Here's how the part is built. I have some questions about the finished solid (model axes, mm). Face numbers are marked on the shaded views. A direction names the side the tool comes from. Round coordinates to 2 decimals unless told otherwise and drop trailing zeros. Write each loop counter-clockwise with the first axis right and the second up, starting at its lowest first coordinate (ties: lowest second). Pieces come first, ordered by that corner, then holes. Notation, with made-up numbers: (47.5, -15.75) - (100.5, -15.75) arc R35 ccw to (100.5, 19.25) - close; hole circle Ø1 at (63.5, -35). An arc over 180 degrees is marked (long way). Write item = value, one per line. Start each with the question number.
Item 1: If I drill on line 1 along Y through (x, z) = (60, 26); line 2 along Y through (x, z) = (75.5, 38); line 3 along Z through (x, y) = (74, -28), over which ranges is the centre line in solid material (lowest first)? Write a range as [from, to].
Item 2: If we section it at B-B (z = -39.5): Please give me the cut outline in (x, y), and give its area (3 significant figures).
Item 3: Which directions (+Z, -Z, +X, -X, +Y, -Y) give clear straight access to the entire face, cutting with the end or side of a thin tool? Please do the marked faces 1, 2 and 3.
Item 4: If we section it at A-A (x = 2): Please give me the cut outline in (y, z).
Item 5: If we section it at C-C (y = -16.5): Please give me the cut outline in (x, z), and give its area (3 significant figures).
Item 6: For P1, Ø8, axis at x = -26, y = 34.5, coming from the -Z side; P2, Ø22, axis at x = 7.5, y = 22, coming from the +Z side; P3, Ø22, axis at x = 5.5, z = -57, coming from the -Y side, each with a flat end and sliding along its axis, tell me the tip position at first contact or that it passes through.
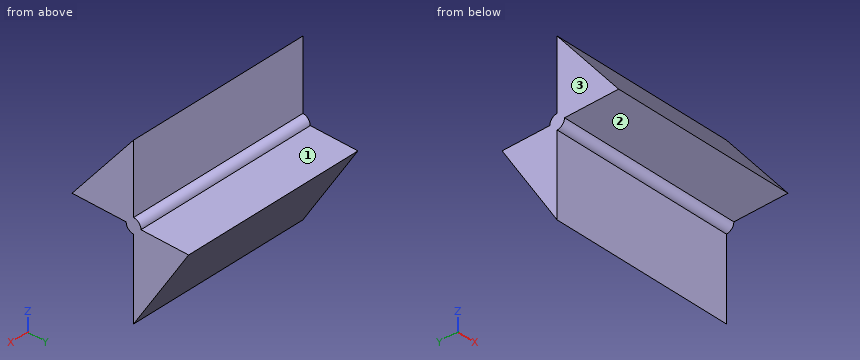
```python
from build123d import *

# Parameters (mm, degrees)
F2_DEPTH      = 115.1771843433
F2_DEPTH_BACK = 52.7988504618


# Not quite as in the source:
# - the program builds the solid bodies; features that only make, move or delete a surface that nothing else refers to are left out


with BuildPart() as f2:
    # F0 (on Right) → F2 (new body, two sides)
    with BuildSketch(Plane.YZ) as f2_sk:
        with BuildLine():
            Line((0, 70.4632103443), (-56.6462948918, 0))
            Line((-56.6462948918, 0), (-6.8218263729, 0))
            ThreePointArc((-6.8218263729, 0), (-4.8237596884, -4.8237596884), (0, -6.8218263729))
            Line((0, -6.8218263729), (0, -80.7569846511))
            Line((0, -80.7569846511), (50.7276728749, 0))
            Line((50.7276728749, 0), (6.8218263729, 0))
            ThreePointArc((6.8218263729, 0), (4.8237596884, 4.8237596884), (0, 6.8218263729))
            Line((0, 6.8218263729), (0, 16.5492296219))
            Line((0, 16.5492296219), (0, 70.4632103443))
        make_face()
    extrude(amount=F2_DEPTH)
    extrude(f2_sk.sketch, amount=-F2_DEPTH_BACK)


solid = f2.part
```
Reply:
q1.line_1 = [-35.74, 0]
q1.line_2 = [-26.1, 0]
q1.line_3 = [0, 35.63]
q2.outline = (-52.8, 0) - (115.18, 0) - (115.18, 25.92) - (-52.8, 25.92) - close
q2.area = 4,350 mm2
q3.face_1 = +Z, +X, -X, +Y
q3.face_2 = -Z, +X, -X, -Y
q3.face_3 = +Z, -Z, -X, +Y, -Y
q4.outline = (-56.65, 0) - (-6.82, 0) arc R6.82 ccw to (0, -6.82) - (0, -80.76) - (50.73, 0) - (6.82, 0) arc R6.82 ccw to (0, 6.82) - (0, 70.46) - close
q5.outline = (-52.8, 0) - (115.18, 0) - (115.18, 49.94) - (-52.8, 49.94) - close
q5.area = 8,390 mm2
q6.P1 = -32.2
q6.P2 = 0
q6.P3 = 0
